Solid Edge part; units mm, degrees
sketch "Sketch1" plane through (0, 0, 0) normal (0, 0, 1) x (1, 0, 0)
  line L0 (-30, -5) -> (30, -5)
  line L1 (30, -5) -> (30, 5)
  line L2 (30, 5) -> (-30, 5)
  line L3 (-30, 5) -> (-30, -5)
  dimension "D1" = 30
  dimension "D2" = 30
extrude "Protrusion1" add sketch "Sketch1" along normal mid plane 74
sketch "Sketch2" plane through (0, 0, 37) normal (0, 0, 1) x (1, 0, 0)
  circle A0 centre (-20, 0) radius 1
  circle A1 centre (20, 0) radius 1
extrude "Extrusionsausschnitt_1" cut sketch "Sketch2" against normal blind 15
mirror "Mirror1" about plane through (0, 0, 0) normal (0, 0, 1) of "Extrusionsausschnitt_1"
sketch "Sketch3" plane through (0, -5, 0) normal (0, -1, 0) x (1, 0, 0)
  circle A0 centre (0, 0) radius 11
  circle A1 centre (-15.5, 15.5) radius 1.6
  circle A2 centre (-15.5, -15.5) radius 1.6
  circle A3 centre (15.5, -15.5) radius 1.6
  circle A4 centre (15.5, 15.5) radius 1.6
extrude "Cutout1" cut sketch "Sketch3" against normal through all
properties material "Nylon, allgemein"
CAD build for the part. Positions are in the model's coordinates, mm. A direction names the side the tool comes from. Coordinates: 2 decimals unless noted, no trailing zeros. Order: outer loops, then holes, each group sorted by start corner. A loop starts at its lowest first (then second) coordinate and runs counter-clockwise, first axis right, second up. Notation, with made-up numbers: (13, 12) -> (59, 12) arc R14 ccw to (59, 21) -> close; hole circle Ø4 at (55.5, 51). An arc over 180 degrees is marked (long way). Answer in a Markdown table with one row per item.
1) Drill centre lines: line 1 (Z direction, x = -15.5, y = -2); line 2 (Z direction, x = 0, y = 2); line 3 (X direction, y = 0.25, z = 31). Where is each one in solid material? Low to high.
Check values:
| item | result |
|---|---|
| line 1 | -37 to -17.1, -13.9 to 13.9, 17.1 to 37 |
| line 2 | -37 to -11, 11 to 37 |
| line 3 | -30 to -20.97, -19.03 to 19.03, 20.97 to 30 |
2) Band-saw the part on D-D (z = 0). List the corners of the cut face in (x, y), and give its area (3 significant figures).
Check values:
| item | result |
|---|---|
| outline | (-30, -5) -> (-11, -5) -> (-11, 5) -> (-30, 5) -> close; (11, -5) -> (30, -5) -> (30, 5) -> (11, 5) -> close |
| area | 380 mm2 |
3) Band-saw the part on C-C (y = 0). List the corners of the cut face in (x, z), and give its area (3 significant figures).
Check values:
| item | result |
|---|---|
| outline | (-30, -37) -> (-21, -37) -> (-21, -22) -> (-19, -22) -> (-19, -37) -> (19, -37) -> (19, -22) -> (21, -22) -> (21, -37) -> (30, -37) -> (30, 37) -> (21, 37) -> (21, 22) -> (19, 22) -> (19, 37) -> (-19, 37) -> (-19, 22) -> (-21, 22) -> (-21, 37) -> (-30, 37) -> close; hole circle Ø3.2 at (-15.5, -15.5); hole circle Ø3.2 at (-15.5, 15.5); hole circle Ø22 at (0, 0); hole circle Ø3.2 at (15.5, -15.5); hole circle Ø3.2 at (15.5, 15.5) |
| area | 3,910 mm2 |
4) Mould opens along Y. For faces 1 (the face through (7, 5, -9)), 2 (the face through (-16.68, -0.07, 16.58)), 3 (the face through (-20, 0, -22)), 4 (the face through (-21, 0, -30)) say: pulls with the +Y half, pulls with the -Y half, needs draft (parallel to the pull), parting line crosses it, or undercut.
Check values:
| item | result |
|---|---|
| face 1 | pulls with the +Y half |
| face 2 | needs draft |
| face 3 | undercut |
| face 4 | undercut |
5) Band-saw the part on B-B (x = 0). List the corners of the cut face in (y, z).
Check values:
| item | result |
|---|---|
| outline | (-5, -37) -> (5, -37) -> (5, -11) -> (-5, -11) -> close; (-5, 11) -> (5, 11) -> (5, 37) -> (-5, 37) -> close |
6) Flat gauge pins, fed straight in: P1, Ø1.8, axis at x = -20, y = 0, coming from the -Z side; P2, Ø1, axis at x = 20, y = 0, coming from the +Z side; P3, Ø1.9, axis at x = 15.5, z = -15.5, coming from the -Y side. Where does each tip first touch, or does it go through?
Check values:
| item | result |
|---|---|
| P1 | z = -22 |
| P2 | z = 22 |
| P3 | through |
7) Band-saw the part on A-A (z = -15.5). List the corners of the cut face in (x, y), and give its area (3 significant figures).
Check values:
| item | result |
|---|---|
| outline | (-30, -5) -> (-17.1, -5) -> (-17.1, 5) -> (-30, 5) -> close; (-13.9, -5) -> (13.9, -5) -> (13.9, 5) -> (-13.9, 5) -> close; (17.1, -5) -> (30, -5) -> (30, 5) -> (17.1, 5) -> close |
| area | 536 mm2 |
8) Which spindle directions (+Z, -Z, +X, -X, +Y, -Y) get a long thin tool onto all of the face, cutting with end or side? Do faces 5 (the face through (-16.68, -0.07, -14.42)), 6 (the face through (19, 0, -30)), 7 (the face through (-20, 0, 22)). Say none if no direction does.
Check values:
| item | result |
|---|---|
| face 5 | +Y, -Y |
| face 6 | -Z |
| face 7 | +Z |
